CAD build for the part. Positions are in the model's coordinates, mm. Face numbers are marked on the shaded views. A direction names the side the tool comes from. Give positions to 0.01 mm unless a question says otherwise; leave off trailing zeros. Order: outer loops, then holes, each group sorted by start corner. A loop starts at its lowest first (then second) coordinate and runs counter-clockwise, first axis right, second up. Notation, with made-up numbers: M -10,-1 L 13,-1 A14 cw 13,26 Z; hole C 84,54 d7. An arc over 180 degrees is marked long. Put each result on its own line as item: value. Start each with the question number.
1) Drill centre lines: line 1 (X direction, y = -14.6, z = 40); line 2 (X direction, y = -4, z = 127); line 3 (Y direction, x = 8.5, z = 17.5). Where is each one in solid material? Low to high. Write a range as [from, to].
2) Tool access for the marked faces 1 and 2: list every direction of +Z, -Z, +X, -X, +Y, -Y with a clear straight run to the whole face (end or side of a thin tool).
3) Two-plate mould, pull along Y, no slides. Class the marked faces 3, 4 and 5: released by +Y, released by -Y, zero draft, split by the parting line, or undercut.
4) Cut at D-D (z = 144.5). Write the cut outline in (x, y).
5) Cut at A-A (z = 20). Give the number of separate pieces and of enclosed holes in the cut face, and give its area (3 significant figures).
6) Pin check, flat tip, straight feed: pin 1 (8 mm diameter, centred on x = 0.5, y = -7, fed in from -Z). Stop position of the tip, or through.
7) Cut at C-C (z = 117.5). Write the cut outline in (x, y), and give its area (3 significant figures).
8) Cut at B-B (y = 0). Write the cut outline in (x, z), and give its area (4 significant figures).
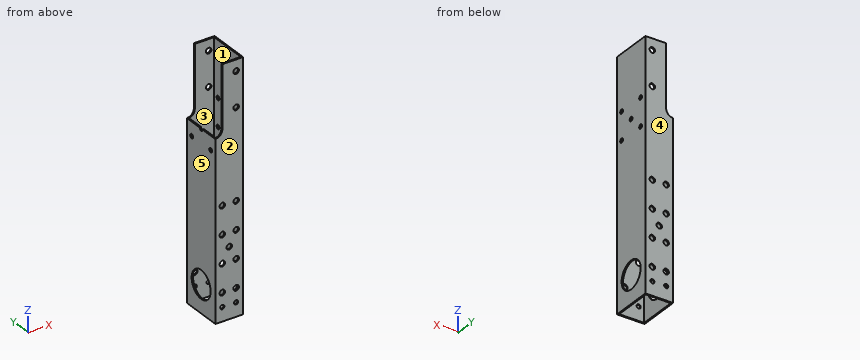
```python
from build123d import *

# Parameters (mm, degrees)
SKETCH_1_W          = 20
SKETCH_1_H          = 30
SKETCH_1_W_2        = 18
SKETCH_1_H_2        = 28
EXTRUDE_1_DEPTH     = 177.5
CUT_EXTRUDE_1_REACH = 182.295
SKETCH_2_R          = 1.5
CUT_EXTRUDE_2_REACH = 182.295
SKETCH_3_W          = 5
SKETCH_3_H          = 50
FILLET_1_R          = 5
CUT_EXTRUDE_3_REACH = 182.295
SKETCH_4_R          = 2
CUT_EXTRUDE_4_REACH = 182.295
SKETCH_5_R          = 2
CUT_EXTRUDE_5_REACH = 181.252
SKETCH_6_R          = 1.5
SKETCH_6_R_2        = 10


with BuildPart() as part:
    # 草图1 → 拉伸-薄壁1 (new body)
    with BuildSketch(Plane.XY):
        Rectangle(SKETCH_1_W, SKETCH_1_H)
        Rectangle(SKETCH_1_W_2, SKETCH_1_H_2, mode=Mode.SUBTRACT)
    extrude(amount=EXTRUDE_1_DEPTH)

    # 切除-拉伸1: up to this face of the body (flat: up to its plane)
    cut_extrude_1_end = Plane(part.part.faces().sort_by_distance((0, -15, 88.75))[0])
    # 草图2 → 切除-拉伸1 (cut, up to the picked face)
    with BuildSketch(Plane(origin=(0, 15, 0), x_dir=(1, 0, 0), z_dir=(0, 1, 0)), mode=Mode.PRIVATE) as cut_extrude_1_sk1:
        with Locations(Location((5, -10, 0), (0, 0, 270))):
            Circle(SKETCH_2_R)
    cut_extrude_1_tool1 = split(extrude(cut_extrude_1_sk1.sketch, amount=-CUT_EXTRUDE_1_REACH, mode=Mode.PRIVATE), bisect_by=cut_extrude_1_end, keep=Keep.BOTH, mode=Mode.PRIVATE)
    # 草图2 → 切除-拉伸1 (cut, up to the picked face)
    with BuildSketch(Plane(origin=(0, 15, 0), x_dir=(1, 0, 0), z_dir=(0, 1, 0)), mode=Mode.PRIVATE) as cut_extrude_1_sk2:
        with Locations(Location((-5, -10, 0), (0, 0, 270))):
            Circle(SKETCH_2_R)
    cut_extrude_1_tool2 = split(extrude(cut_extrude_1_sk2.sketch, amount=-CUT_EXTRUDE_1_REACH, mode=Mode.PRIVATE), bisect_by=cut_extrude_1_end, keep=Keep.BOTH, mode=Mode.PRIVATE)
    add(cut_extrude_1_tool1.solids().sort_by(Axis((5, 15, 10), (0, -1, 0)))[0], mode=Mode.SUBTRACT)
    add(cut_extrude_1_tool2.solids().sort_by(Axis((-5, 15, 10), (0, -1, 0)))[0], mode=Mode.SUBTRACT)

    # 切除-拉伸2: up to this face of the body (flat: up to its plane)
    cut_extrude_2_end = Plane(part.part.faces().sort_by_distance((0, -15, 89.064860035))[0])
    # 草图3 → 切除-拉伸2 (cut, up to the picked face)
    with BuildSketch(Plane(origin=(0, 15, 0), x_dir=(1, 0, 0), z_dir=(0, 1, 0)), mode=Mode.PRIVATE) as cut_extrude_2_sk1:
        with Locations((-7.5, -152.5)):
            Rectangle(SKETCH_3_W, SKETCH_3_H)
    cut_extrude_2_tool1 = split(extrude(cut_extrude_2_sk1.sketch, amount=-CUT_EXTRUDE_2_REACH, mode=Mode.PRIVATE), bisect_by=cut_extrude_2_end, keep=Keep.BOTH, mode=Mode.PRIVATE)
    add(cut_extrude_2_tool1.solids().sort_by(Axis((-7.5, 15, 152.5), (0, -1, 0)))[0], mode=Mode.SUBTRACT)

    # 圆角1
    fillet_1_edges = [part.edges().sort_by_distance(p)[0] for p in [
        (-5, 14.5, 127.5),
    ]]
    fillet(fillet_1_edges, radius=FILLET_1_R - 0.0001)  # a hair under: the kernel refuses the full size

    # 切除-拉伸3: up to this face of the body (flat: up to its plane)
    cut_extrude_3_end = Plane(part.part.faces().sort_by_distance((0.559725578, -15, 84.310829926))[0])
    # 草图4 → 切除-拉伸3 (cut, up to the picked face)
    with BuildSketch(Plane(origin=(0, 15, 0), x_dir=(1, 0, 0), z_dir=(0, 1, 0)), mode=Mode.PRIVATE) as cut_extrude_3_sk1:
        with Locations(Location((5, -144.5, 0), (0, 0, 270))):
            Circle(SKETCH_4_R)
    cut_extrude_3_tool1 = split(extrude(cut_extrude_3_sk1.sketch, amount=-CUT_EXTRUDE_3_REACH, mode=Mode.PRIVATE), bisect_by=cut_extrude_3_end, keep=Keep.BOTH, mode=Mode.PRIVATE)
    # 草图4 → 切除-拉伸3 (cut, up to the picked face)
    with BuildSketch(Plane(origin=(0, 15, 0), x_dir=(1, 0, 0), z_dir=(0, 1, 0)), mode=Mode.PRIVATE) as cut_extrude_3_sk2:
        with Locations(Location((5, -169.5, 0), (0, 0, 270))):
            Circle(SKETCH_4_R)
    cut_extrude_3_tool2 = split(extrude(cut_extrude_3_sk2.sketch, amount=-CUT_EXTRUDE_3_REACH, mode=Mode.PRIVATE), bisect_by=cut_extrude_3_end, keep=Keep.BOTH, mode=Mode.PRIVATE)
    add(cut_extrude_3_tool1.solids().sort_by(Axis((5, 15, 144.5), (0, -1, 0)))[0], mode=Mode.SUBTRACT)
    add(cut_extrude_3_tool2.solids().sort_by(Axis((5, 15, 169.5), (0, -1, 0)))[0], mode=Mode.SUBTRACT)

    # 切除-拉伸4: up to this face of the body (flat: up to its plane)
    cut_extrude_4_end = Plane(part.part.faces().sort_by_distance((0.525557475, 15, 83.751483629))[0])
    # 草图5 → 切除-拉伸4 (cut, up to the picked face)
    with BuildSketch(Plane.XZ.offset(15), mode=Mode.PRIVATE) as cut_extrude_4_sk1:
        with Locations(Location((5, 20, 0), (0, 0, 270))):
            Circle(SKETCH_5_R)
    cut_extrude_4_tool1 = split(extrude(cut_extrude_4_sk1.sketch, amount=-CUT_EXTRUDE_4_REACH, mode=Mode.PRIVATE), bisect_by=cut_extrude_4_end, keep=Keep.BOTH, mode=Mode.PRIVATE)
    # 草图5 → 切除-拉伸4 (cut, up to the picked face)
    with BuildSketch(Plane.XZ.offset(15), mode=Mode.PRIVATE) as cut_extrude_4_sk2:
        with Locations(Location((5, 40, 0), (0, 0, 270))):
            Circle(SKETCH_5_R)
    cut_extrude_4_tool2 = split(extrude(cut_extrude_4_sk2.sketch, amount=-CUT_EXTRUDE_4_REACH, mode=Mode.PRIVATE), bisect_by=cut_extrude_4_end, keep=Keep.BOTH, mode=Mode.PRIVATE)
    # 草图5 → 切除-拉伸4 (cut, up to the picked face)
    with BuildSketch(Plane.XZ.offset(15), mode=Mode.PRIVATE) as cut_extrude_4_sk3:
        with Locations(Location((5, 60, 0), (0, 0, 270))):
            Circle(SKETCH_5_R)
    cut_extrude_4_tool3 = split(extrude(cut_extrude_4_sk3.sketch, amount=-CUT_EXTRUDE_4_REACH, mode=Mode.PRIVATE), bisect_by=cut_extrude_4_end, keep=Keep.BOTH, mode=Mode.PRIVATE)
    # 草图5 → 切除-拉伸4 (cut, up to the picked face)
    with BuildSketch(Plane.XZ.offset(15), mode=Mode.PRIVATE) as cut_extrude_4_sk4:
        with Locations(Location((5, 80, 0), (0, 0, 270))):
            Circle(SKETCH_5_R)
    cut_extrude_4_tool4 = split(extrude(cut_extrude_4_sk4.sketch, amount=-CUT_EXTRUDE_4_REACH, mode=Mode.PRIVATE), bisect_by=cut_extrude_4_end, keep=Keep.BOTH, mode=Mode.PRIVATE)
    # 草图5 → 切除-拉伸4 (cut, up to the picked face)
    with BuildSketch(Plane.XZ.offset(15), mode=Mode.PRIVATE) as cut_extrude_4_sk5:
        with Locations(Location((-5, 80, 0), (0, 0, 270))):
            Circle(SKETCH_5_R)
    cut_extrude_4_tool5 = split(extrude(cut_extrude_4_sk5.sketch, amount=-CUT_EXTRUDE_4_REACH, mode=Mode.PRIVATE), bisect_by=cut_extrude_4_end, keep=Keep.BOTH, mode=Mode.PRIVATE)
    # 草图5 → 切除-拉伸4 (cut, up to the picked face)
    with BuildSketch(Plane.XZ.offset(15), mode=Mode.PRIVATE) as cut_extrude_4_sk6:
        with Locations(Location((-5, 60, 0), (0, 0, 270))):
            Circle(SKETCH_5_R)
    cut_extrude_4_tool6 = split(extrude(cut_extrude_4_sk6.sketch, amount=-CUT_EXTRUDE_4_REACH, mode=Mode.PRIVATE), bisect_by=cut_extrude_4_end, keep=Keep.BOTH, mode=Mode.PRIVATE)
    # 草图5 → 切除-拉伸4 (cut, up to the picked face)
    with BuildSketch(Plane.XZ.offset(15), mode=Mode.PRIVATE) as cut_extrude_4_sk7:
        with Locations(Location((-5, 40, 0), (0, 0, 270))):
            Circle(SKETCH_5_R)
    cut_extrude_4_tool7 = split(extrude(cut_extrude_4_sk7.sketch, amount=-CUT_EXTRUDE_4_REACH, mode=Mode.PRIVATE), bisect_by=cut_extrude_4_end, keep=Keep.BOTH, mode=Mode.PRIVATE)
    # 草图5 → 切除-拉伸4 (cut, up to the picked face)
    with BuildSketch(Plane.XZ.offset(15), mode=Mode.PRIVATE) as cut_extrude_4_sk8:
        with Locations(Location((-5, 20, 0), (0, 0, 270))):
            Circle(SKETCH_5_R)
    cut_extrude_4_tool8 = split(extrude(cut_extrude_4_sk8.sketch, amount=-CUT_EXTRUDE_4_REACH, mode=Mode.PRIVATE), bisect_by=cut_extrude_4_end, keep=Keep.BOTH, mode=Mode.PRIVATE)
    # 草图5 → 切除-拉伸4 (cut, up to the picked face)
    with BuildSketch(Plane.XZ.offset(15), mode=Mode.PRIVATE) as cut_extrude_4_sk9:
        with Locations(Location((0, 50, 0), (0, 0, 270))):
            Circle(SKETCH_5_R)
    cut_extrude_4_tool9 = split(extrude(cut_extrude_4_sk9.sketch, amount=-CUT_EXTRUDE_4_REACH, mode=Mode.PRIVATE), bisect_by=cut_extrude_4_end, keep=Keep.BOTH, mode=Mode.PRIVATE)
    add(cut_extrude_4_tool1.solids().sort_by(Axis((5, -15, 20), (0, 1, 0)))[0], mode=Mode.SUBTRACT)
    add(cut_extrude_4_tool2.solids().sort_by(Axis((5, -15, 40), (0, 1, 0)))[0], mode=Mode.SUBTRACT)
    add(cut_extrude_4_tool3.solids().sort_by(Axis((5, -15, 60), (0, 1, 0)))[0], mode=Mode.SUBTRACT)
    add(cut_extrude_4_tool4.solids().sort_by(Axis((5, -15, 80), (0, 1, 0)))[0], mode=Mode.SUBTRACT)
    add(cut_extrude_4_tool5.solids().sort_by(Axis((-5, -15, 80), (0, 1, 0)))[0], mode=Mode.SUBTRACT)
    add(cut_extrude_4_tool6.solids().sort_by(Axis((-5, -15, 60), (0, 1, 0)))[0], mode=Mode.SUBTRACT)
    add(cut_extrude_4_tool7.solids().sort_by(Axis((-5, -15, 40), (0, 1, 0)))[0], mode=Mode.SUBTRACT)
    add(cut_extrude_4_tool8.solids().sort_by(Axis((-5, -15, 20), (0, 1, 0)))[0], mode=Mode.SUBTRACT)
    add(cut_extrude_4_tool9.solids().sort_by(Axis((0, -15, 50), (0, 1, 0)))[0], mode=Mode.SUBTRACT)

    # 切除-拉伸5: up to this face of the body (flat: up to its plane)
    cut_extrude_5_end = Plane(part.part.faces().sort_by_distance((-10, 0, 63.75))[0])
    # 草图6 → 切除-拉伸5 (cut, up to the picked face)
    with BuildSketch(Plane(origin=(10, 0, 0), x_dir=(0, 0, -1), z_dir=(1, 0, 0)), mode=Mode.PRIVATE) as cut_extrude_5_sk1:
        with Locations((-127.5, 0)):
            Circle(SKETCH_6_R)
    cut_extrude_5_tool1 = split(extrude(cut_extrude_5_sk1.sketch, amount=-CUT_EXTRUDE_5_REACH, mode=Mode.PRIVATE), bisect_by=cut_extrude_5_end, keep=Keep.BOTH, mode=Mode.PRIVATE)
    # 草图6 → 切除-拉伸5 (cut, up to the picked face)
    with BuildSketch(Plane(origin=(10, 0, 0), x_dir=(0, 0, -1), z_dir=(1, 0, 0)), mode=Mode.PRIVATE) as cut_extrude_5_sk2:
        with Locations((-117.5, 10)):
            Circle(SKETCH_6_R)
    cut_extrude_5_tool2 = split(extrude(cut_extrude_5_sk2.sketch, amount=-CUT_EXTRUDE_5_REACH, mode=Mode.PRIVATE), bisect_by=cut_extrude_5_end, keep=Keep.BOTH, mode=Mode.PRIVATE)
    # 草图6 → 切除-拉伸5 (cut, up to the picked face)
    with BuildSketch(Plane(origin=(10, 0, 0), x_dir=(0, 0, -1), z_dir=(1, 0, 0)), mode=Mode.PRIVATE) as cut_extrude_5_sk3:
        with Locations((-117.5, -10)):
            Circle(SKETCH_6_R)
    cut_extrude_5_tool3 = split(extrude(cut_extrude_5_sk3.sketch, amount=-CUT_EXTRUDE_5_REACH, mode=Mode.PRIVATE), bisect_by=cut_extrude_5_end, keep=Keep.BOTH, mode=Mode.PRIVATE)
    # 草图6 → 切除-拉伸5 (cut, up to the picked face)
    with BuildSketch(Plane(origin=(10, 0, 0), x_dir=(0, 0, -1), z_dir=(1, 0, 0)), mode=Mode.PRIVATE) as cut_extrude_5_sk4:
        with Locations((-137.5, -10)):
            Circle(SKETCH_6_R)
    cut_extrude_5_tool4 = split(extrude(cut_extrude_5_sk4.sketch, amount=-CUT_EXTRUDE_5_REACH, mode=Mode.PRIVATE), bisect_by=cut_extrude_5_end, keep=Keep.BOTH, mode=Mode.PRIVATE)
    # 草图6 → 切除-拉伸5 (cut, up to the picked face)
    with BuildSketch(Plane(origin=(10, 0, 0), x_dir=(0, 0, -1), z_dir=(1, 0, 0)), mode=Mode.PRIVATE) as cut_extrude_5_sk5:
        with Locations((-137.5, 10)):
            Circle(SKETCH_6_R)
    cut_extrude_5_tool5 = split(extrude(cut_extrude_5_sk5.sketch, amount=-CUT_EXTRUDE_5_REACH, mode=Mode.PRIVATE), bisect_by=cut_extrude_5_end, keep=Keep.BOTH, mode=Mode.PRIVATE)
    # 草图6 → 切除-拉伸5 (cut, up to the picked face)
    with BuildSketch(Plane(origin=(10, 0, 0), x_dir=(0, 0, -1), z_dir=(1, 0, 0)), mode=Mode.PRIVATE) as cut_extrude_5_sk6:
        with Locations((-20, 0)):
            Circle(SKETCH_6_R_2)
    cut_extrude_5_tool6 = split(extrude(cut_extrude_5_sk6.sketch, amount=-CUT_EXTRUDE_5_REACH, mode=Mode.PRIVATE), bisect_by=cut_extrude_5_end, keep=Keep.BOTH, mode=Mode.PRIVATE)
    add(cut_extrude_5_tool1.solids().sort_by(Axis((10, 0, 127.5), (-1, 0, 0)))[0], mode=Mode.SUBTRACT)
    add(cut_extrude_5_tool2.solids().sort_by(Axis((10, 10, 117.5), (-1, 0, 0)))[0], mode=Mode.SUBTRACT)
    add(cut_extrude_5_tool3.solids().sort_by(Axis((10, -10, 117.5), (-1, 0, 0)))[0], mode=Mode.SUBTRACT)
    add(cut_extrude_5_tool4.solids().sort_by(Axis((10, -10, 137.5), (-1, 0, 0)))[0], mode=Mode.SUBTRACT)
    add(cut_extrude_5_tool5.solids().sort_by(Axis((10, 10, 137.5), (-1, 0, 0)))[0], mode=Mode.SUBTRACT)
    add(cut_extrude_5_tool6.solids().sort_by(Axis((10, 0, 20), (-1, 0, 0)))[0], mode=Mode.SUBTRACT)


solid = part.part
```
Solution:
1. line 1: [-10, -7], [-3, 3], [7, 10]
1. line 2: [-10, -9], [9, 10]
1. line 3: [-15, -14], [14, 15]
2. face 1: +Z, -Z
2. face 2: +Z, -Z, +X, -X, -Y
3. face 3: undercut
3. face 4: released by +Y
3. face 5: zero draft
4. outline: M -5,-15 L 3,-15 L 3,-14 L -5,-14 Z; M -5,14 L 3,14 L 3,15 L -5,15 Z; M 7,-15 L 10,-15 L 10,15 L 7,15 L 7,14 L 9,14 L 9,-14 L 7,-14 Z
5. separate pieces: 6
5. enclosed holes: 0
5. area: 40.0 mm²
6. pin 1: through
7. outline: M -10,-15 L 10,-15 L 10,-11.5 L 9,-11.5 L 9,-14 L -9,-14 L -9,-11.5 L -10,-11.5 Z; M -10,-8.5 L -9,-8.5 L -9,8.5 L -10,8.5 Z; M -10,11.5 L -9,11.5 L -9,14 L 9,14 L 9,11.5 L 10,11.5 L 10,15 L -10,15 Z; M 9,-8.5 L 10,-8.5 L 10,8.5 L 9,8.5 Z
7. area: 84.0 mm²
8. outline: M -10,0 L -9,0 L -9,10 L -10,10 Z; M -10,30 L -9,30 L -9,126 L -10,126 Z; M 9,0 L 10,0 L 10,10 L 9,10 Z; M 9,30 L 10,30 L 10,126 L 9,126 Z; M 9,129 L 10,129 L 10,177.5 L 9,177.5 Z
8. area: 260.5 mm²
